Can you work these out from the model? Positions are in its coordinate system, mm. Face numbers are marked on the shaded views. A direction names the side the tool comes from. Coordinates: 2 decimals unless noted, no trailing zeros. Order: outer loops, then holes, each group sorted by start corner. A loop starts at its lowest first (then second) coordinate and runs counter-clockwise, first axis right, second up. Notation, with made-up numbers: (13.25, 50) -> (21.25, 50) arc R30 ccw to (21.25, 81) -> close; hole circle Ø11 at (61, -0.5). An arc over 180 degrees is marked (long way). Answer in a Markdown table with one row per item. Add a question column.
1. Imagine slicing it at D-D on z = 5. Write out the boundary of the cut face in (x, y).
2. Imagine slicing it at C-C on x = 70. Write out the boundary of the cut face in (y, z), plus the area to 3 significant figures.
3. Will these pins go through, and if not, where does the flat tip stop? pin 1 (12 mm diameter, centred on x = 70, z = -4.28, fed in from -Y); pin 2 (3 mm diameter, centred on y = 32, z = 1, fed in from -X); pin 3 (5 mm diameter, centred on x = 52.5, z = 5.5, fed in from +Y); pin 4 (12 mm diameter, centred on y = 11.5, z = 7.5, fed in from -X).
4. On a 3-axis mill with a long thin cutter (end or side, diameter ignored), from which of +Z, -Z, +X, -X, +Y, -Y can I reach the whole of each face in a straight line? I mean the marked faces 1 and 2. Say none if no direction works.
5. Imagine slicing it at A-A on x = 28.5. Write out the boundary of the cut face in (y, z).
6. Imagine slicing it at B-B on z = -4.28. Write out the boundary of the cut face in (x, y).
7. If I drill on line 1 along Z through (x, y) = (70, 83.75); line 2 along Y through (x, z) = (27.5, -5.25); line 3 along X through (y, z) = (33, 10.5), over which ranges is the centre line in solid material (lowest first)? Write a range as [from, to].
8. We'd pull the mould along Y, two halves only. Please class the marked faces 3, 4 and 5: pulls with the +Y half, pulls with the -Y half, needs draft (parallel to the pull), parting line crosses it, or undercut.
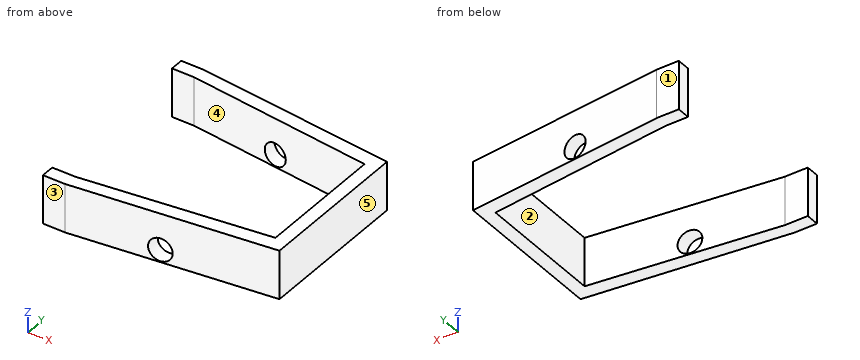
from build123d import *

# Parameters (mm, degrees)
SKETCH042_R      = 5.177463
EXTRUDE045_DEPTH = 800
EXTRUDE044_DEPTH = 22


with BuildPart() as extrude045:
    # Sketch042 → Extrude045 (new body)
    with BuildSketch(Plane.XZ):
        with Locations((70, 3.62)):
            Circle(SKETCH042_R)
    extrude(amount=EXTRUDE045_DEPTH)


with BuildPart() as extrude045_1:
    # Extrude045 placement: moved
    add(extrude045.part.moved(Location((0, 293, 0))))


with BuildPart() as obj1:
    # Sketch041 → Extrude044 (new body)
    with BuildSketch(Plane.XY):
        Polygon((30, 0), (120, 10), (120, 80), (30, 90), (20, 90), (20, 84), (30, 84), (114, 74), (114, 16), (30.22679, 6), (20, 6), (20, 0), align=None)
    extrude(amount=EXTRUDE044_DEPTH)


with BuildPart() as obj1_1:
    # Extrude044 placement: moved
    add(obj1.part.moved(Location((0, 0, -2))))

    # Cut014: cut Extrude045
    add(extrude045_1.part, mode=Mode.SUBTRACT)


with BuildPart() as obj1_2:
    # Cut014 placement: moved
    add(obj1_1.part.moved(Location((0, 0, -7.9))))


solid = obj1_2.part
Answers follow:
| question | item | result |
|---|---|---|
| 1 | outline | (20, 0) -> (30, 0) -> (120, 10) -> (120, 80) -> (30, 90) -> (20, 90) -> (20, 84) -> (30, 84) -> (114, 74) -> (114, 16) -> (30.23, 6) -> (20, 6) -> close |
| 2 | outline | (4.44, -9.9) -> (10.75, -9.9) -> (10.75, -9.46) -> (4.44, -9.46) -> close; (4.44, 0.9) -> (10.75, 0.9) -> (10.75, 12.1) -> (4.44, 12.1) -> close; (79.24, -9.9) -> (85.56, -9.9) -> (85.56, -9.46) -> (79.24, -9.46) -> close; (79.24, 0.9) -> (85.56, 0.9) -> (85.56, 12.1) -> (79.24, 12.1) -> close |
| 2 | area | 147 mm² |
| 3 | pin 1 | stops at y = 3.78 |
| 3 | pin 2 | stops at x = 114 |
| 3 | pin 3 | stops at y = 87.78 |
| 3 | pin 4 | stops at x = 20 |
| 4 | face 1 | +Z, -Z, +X, -X, +Y |
| 4 | face 2 | +Z, -Z, -X |
| 5 | outline | (0, -9.9) -> (6, -9.9) -> (6, 12.1) -> (0, 12.1) -> close; (84, -9.9) -> (90, -9.9) -> (90, 12.1) -> (84, 12.1) -> close |
| 6 | outline | (20, 0) -> (30, 0) -> (64.82, 3.87) -> (64.82, 10.13) -> (30.23, 6) -> (20, 6) -> close; (20, 84) -> (30, 84) -> (64.82, 79.85) -> (64.82, 86.13) -> (30, 90) -> (20, 90) -> close; (75.18, 5.02) -> (120, 10) -> (120, 80) -> (75.18, 84.98) -> (75.18, 78.62) -> (114, 74) -> (114, 16) -> (75.18, 11.37) -> close |
| 7 | line 1 | z = [-9.9, -9.46], [0.9, 12.1] |
| 7 | line 2 | y = [0, 6], [84, 90] |
| 7 | line 3 | x = [114, 120] |
| 8 | face 3 | pulls with the -Y half |
| 8 | face 4 | undercut |
| 8 | face 5 | needs draft |
